```python
from build123d import *

# Parameters (mm, degrees)
SKETCH_1_W              = 10
SKETCH_1_H              = 10
EXTRUDE_1_DEPTH         = 17.5
HOLE_WIZARD_4_1_4_1_1_D = 4.1
HOLE_WIZARD_4_1_4_1_2_D = 4.1
HOLE_WIZARD_M4_1_REACH  = 37.707
HOLE_WIZARD_M4_1_BORE_R = 1.65
HOLE_WIZARD_M4_2_REACH  = 37.707
HOLE_WIZARD_M4_2_BORE_R = 1.65
CHAMFER_1_SIZE          = 0.3


with BuildPart() as part:
    # 草图1 → 凸台-拉伸1 (new, symmetric)
    with BuildSketch(Plane.XY):
        Rectangle(SKETCH_1_W, SKETCH_1_H)
    extrude(amount=EXTRUDE_1_DEPTH, both=True)

    # Ø4.1 (4.1) 直径孔1 (through all)
    with Locations(Plane(origin=(5, 0, 0), x_dir=(0, 0, -1), z_dir=(1, 0, 0))):
        with Locations((-10, 0), (10, 0)):
            Hole(HOLE_WIZARD_4_1_4_1_1_D / 2)

    # Ø4.1 (4.1) 直径孔2 (through all)
    with Locations(Plane(origin=(0, 5, 0), x_dir=(1, 0, 0), z_dir=(0, 1, 0))):
        with Locations((0, -10), (0, 10)):
            Hole(HOLE_WIZARD_4_1_4_1_2_D / 2)

    # M4 螺纹孔1 bore → M4 螺纹孔1 (cut, up to next)
    with BuildSketch(Plane.XY.offset(17.5), mode=Mode.PRIVATE) as hole_wizard_m4_1_sk1:
        Circle(HOLE_WIZARD_M4_1_BORE_R)
    hole_wizard_m4_1_tool1 = extrude(hole_wizard_m4_1_sk1.sketch, amount=-HOLE_WIZARD_M4_1_REACH, mode=Mode.PRIVATE) & part.part
    add(hole_wizard_m4_1_tool1.solids().sort_by_distance((0, 0, 17.5))[0], mode=Mode.SUBTRACT)

    # M4 螺纹孔2 bore → M4 螺纹孔2 (cut, up to next)
    with BuildSketch(Plane(origin=(0, 0, -17.5), x_dir=(-1, 0, 0), z_dir=(0, 0, -1)), mode=Mode.PRIVATE) as hole_wizard_m4_2_sk1:
        Circle(HOLE_WIZARD_M4_2_BORE_R)
    hole_wizard_m4_2_tool1 = extrude(hole_wizard_m4_2_sk1.sketch, amount=-HOLE_WIZARD_M4_2_REACH, mode=Mode.PRIVATE) & part.part
    add(hole_wizard_m4_2_tool1.solids().sort_by_distance((0, 0, -17.5))[0], mode=Mode.SUBTRACT)

    # 倒角1
    chamfer_1_edges = [part.edges().sort_by_distance(p)[0] for p in [
        (-5, 0, 17.5),
        (5, 0, -12.05),
        (-5, 0, -12.05),
        (0, -5, 17.5),
        (5, 0, 7.95),
        (-5, 0, 7.95),
        (2.05, -5, -10),
        (2.05, 5, -10),
        (2.05, -5, 10),
        (2.05, 5, 10),
        (5, 0, 17.5),
        (0, -5, -17.5),
        (-5, 0, -17.5),
        (-1.65, 0, 17.5),
        (0, 5, -17.5),
        (5, 0, -17.5),
        (1.65, 0, -17.5),
        (5, -5, 0),
        (-5, -5, 0),
        (-5, 5, 0),
        (5, 5, 0),
        (0, 5, 17.5),
    ]]
    chamfer(chamfer_1_edges, length=CHAMFER_1_SIZE)


solid = part.part
```
Geometry check sheet. Reference: the model listing, model coordinates, mm. Coordinates: 2 decimals unless noted, no trailing zeros. Order: outer loops, then holes, each group sorted by start corner. A loop starts at its lowest first (then second) coordinate and runs counter-clockwise, first axis right, second up. Notation, with made-up numbers: M 1.5,-21 L 22.5,-21 A13 ccw 22.5,-14 Z; hole C 73.25,10.5 d2. An arc over 180 degrees is marked long. Answer as a JSON object with one key per item and string values.
Q1. Scan lines: line 1 (Z direction, x = 0, y = -2.25); line 2 (Z direction, x = 0, y = -1.8); line 3 (Y direction, x = 0, z = 14.05). Record each from-to range of solid material in increasing order.
Results are:
{"line 1": "z = -17.5 to -12.05, -7.95 to 7.95, 12.05 to 17.5", "line 2": "z = -17.35 to -12.05, -7.95 to 7.95, 12.05 to 17.35", "line 3": "y = -5 to -1.65, 1.65 to 5"}
Q2. Depth check by flat-ended pin: pin 1 Ø4.5 at (y, z) = (0, 10) entering from -X; pin 2 Ø4.5 at (x, z) = (0, -10) entering from +Y. Enter the tip coordinate at first touch or a pass-through.
Results are:
{"pin 1": "stops at x = -4.9", "pin 2": "stops at y = 4.9"}
Q3. Cross-section at C-C on z = -14.5. Record the cut outline in (x, y), and give its area (3 significant figures).
Results are:
{"outline": "M -5,-4.7 L -4.7,-5 L 4.7,-5 L 5,-4.7 L 5,4.7 L 4.7,5 L -4.7,5 L -5,4.7 Z; hole C 0,0 d3.3", "area": "91.3 mm²"}
Q4. Cross-section at D-D on y = 0.5. Give the number of separate pieces and of enclosed holes in the cut face, and give its area (3 significant figures).
Results are:
{"separate pieces": "5", "enclosed holes": "0", "area": "235 mm²"}
Q5. Cross-section at A-A on z = -10. Record the cut outline in (x, y), and give its area (3 significant figures).
Results are:
{"outline": "M -5,-4.7 L -4.7,-5 L -2.35,-5 L -2.05,-4.7 L -2.05,-2.05 L -4.7,-2.05 L -5,-2.35 Z; M -5,2.35 L -4.7,2.05 L -2.05,2.05 L -2.05,4.7 L -2.35,5 L -4.7,5 L -5,4.7 Z; M 2.05,-4.7 L 2.35,-5 L 4.7,-5 L 5,-4.7 L 5,-2.35 L 4.7,-2.05 L 2.05,-2.05 Z; M 2.05,2.05 L 4.7,2.05 L 5,2.35 L 5,4.7 L 4.7,5 L 2.35,5 L 2.05,4.7 Z", "area": "34.3 mm²"}
Q6. Cross-section at B-B on x = 3.5. Record the cut outline in (y, z), and give its area (3 significant figures).
Results are:
{"outline": "M -5,-17.2 L -4.7,-17.5 L 4.7,-17.5 L 5,-17.2 L 5,17.2 L 4.7,17.5 L -4.7,17.5 L -5,17.2 Z; hole C 0,-10 d4.1; hole C 0,10 d4.1", "area": "323 mm²"}
Q7. Release check for a two-part mould opening along Z. For faces 1 (the cylindrical face through (2.84, 0.09, 7.95)), 2 (the flat face through (-2.2, 0.1, -17.5)), 3 (the cylindrical face through (-2.91, -0.79, -8.11)), 4 (the flat face through (0, -5, 0)) record: released by +Z, released by -Z, zero draft, split by the parting line, or undercut.
Results are:
{"face 1": "undercut", "face 2": "released by -Z", "face 3": "undercut", "face 4": "zero draft"}
